from build123d import *

# Parameters (mm, degrees)
BOSS_EXTRUDE1_DEPTH = 1219.2
SKETCH3_R           = 4.7625
CUT_EXTRUDE1_DEPTH  = 1.27
SKETCH4_R           = 4.7625
CUT_EXTRUDE2_DEPTH  = 1.27
FILLET1_R           = 3.175
FILLET2_R           = 1.5875
CUT_EXTRUDE3_DEPTH  = 457.2


with BuildPart() as part:
    # Sketch1 → Boss-Extrude1 (new body)
    with BuildSketch(Plane(origin=(0, 0, 0), x_dir=(1, 0, 0), z_dir=(0, 1, 0))):
        Polygon((1.27, 1.27), (1.27, 30.48), (1.27, 31.75), (0, 31.75), (0, 0), (31.75, 0), (31.75, 1.27), (30.48, 1.27), align=None)
    extrude(amount=BOSS_EXTRUDE1_DEPTH)

    # Sketch3 → Cut-Extrude1 (cut)
    with BuildSketch(Plane.ZY):
        with Locations((-17.4625, 12.7)):
            Circle(SKETCH3_R)
        with Locations((-17.4625, 38.1)):
            Circle(SKETCH3_R)
        with Locations((-17.4625, 63.5)):
            Circle(SKETCH3_R)
        with Locations((-17.4625, 88.9)):
            Circle(SKETCH3_R)
        with Locations((-17.4625, 114.3)):
            Circle(SKETCH3_R)
        with Locations((-17.4625, 139.7)):
            Circle(SKETCH3_R)
        with Locations((-17.4625, 165.1)):
            Circle(SKETCH3_R)
        with Locations((-17.4625, 190.5)):
            Circle(SKETCH3_R)
        with Locations((-17.4625, 215.9)):
            Circle(SKETCH3_R)
        with Locations((-17.4625, 241.3)):
            Circle(SKETCH3_R)
        with Locations((-17.4625, 266.7)):
            Circle(SKETCH3_R)
        with Locations((-17.4625, 292.1)):
            Circle(SKETCH3_R)
        with Locations((-17.4625, 317.5)):
            Circle(SKETCH3_R)
        with Locations((-17.4625, 342.9)):
            Circle(SKETCH3_R)
        with Locations((-17.4625, 368.3)):
            Circle(SKETCH3_R)
        with Locations((-17.4625, 393.7)):
            Circle(SKETCH3_R)
        with Locations((-17.4625, 419.1)):
            Circle(SKETCH3_R)
        with Locations((-17.4625, 444.5)):
            Circle(SKETCH3_R)
        with Locations((-17.4625, 469.9)):
            Circle(SKETCH3_R)
        with Locations((-17.4625, 495.3)):
            Circle(SKETCH3_R)
        with Locations((-17.4625, 520.7)):
            Circle(SKETCH3_R)
        with Locations((-17.4625, 546.1)):
            Circle(SKETCH3_R)
        with Locations((-17.4625, 571.5)):
            Circle(SKETCH3_R)
        with Locations((-17.4625, 596.9)):
            Circle(SKETCH3_R)
        with Locations((-17.4625, 622.3)):
            Circle(SKETCH3_R)
        with Locations((-17.4625, 647.7)):
            Circle(SKETCH3_R)
        with Locations((-17.4625, 673.1)):
            Circle(SKETCH3_R)
        with Locations((-17.4625, 698.5)):
            Circle(SKETCH3_R)
        with Locations((-17.4625, 723.9)):
            Circle(SKETCH3_R)
        with Locations((-17.4625, 749.3)):
            Circle(SKETCH3_R)
        with Locations((-17.4625, 774.7)):
            Circle(SKETCH3_R)
        with Locations((-17.4625, 800.1)):
            Circle(SKETCH3_R)
        with Locations((-17.4625, 825.5)):
            Circle(SKETCH3_R)
        with Locations((-17.4625, 850.9)):
            Circle(SKETCH3_R)
        with Locations((-17.4625, 876.3)):
            Circle(SKETCH3_R)
        with Locations((-17.4625, 901.7)):
            Circle(SKETCH3_R)
        with Locations((-17.4625, 927.1)):
            Circle(SKETCH3_R)
        with Locations((-17.4625, 952.5)):
            Circle(SKETCH3_R)
        with Locations((-17.4625, 977.9)):
            Circle(SKETCH3_R)
        with Locations((-17.4625, 1003.3)):
            Circle(SKETCH3_R)
        with Locations((-17.4625, 1028.7)):
            Circle(SKETCH3_R)
        with Locations((-17.4625, 1054.1)):
            Circle(SKETCH3_R)
        with Locations((-17.4625, 1079.5)):
            Circle(SKETCH3_R)
        with Locations((-17.4625, 1104.9)):
            Circle(SKETCH3_R)
        with Locations((-17.4625, 1130.3)):
            Circle(SKETCH3_R)
        with Locations((-17.4625, 1155.7)):
            Circle(SKETCH3_R)
        with Locations((-17.4625, 1181.1)):
            Circle(SKETCH3_R)
        with Locations((-17.4625, 1206.5)):
            Circle(SKETCH3_R)
    extrude(amount=-CUT_EXTRUDE1_DEPTH, mode=Mode.SUBTRACT)

    # Sketch4 → Cut-Extrude2 (cut)
    with BuildSketch(Plane.XY):
        with Locations((17.4625, 1206.5)):
            Circle(SKETCH4_R)
        with Locations((17.4625, 1181.1)):
            Circle(SKETCH4_R)
        with Locations((17.4625, 1155.7)):
            Circle(SKETCH4_R)
        with Locations((17.4625, 1130.3)):
            Circle(SKETCH4_R)
        with Locations((17.4625, 1104.9)):
            Circle(SKETCH4_R)
        with Locations((17.4625, 1079.5)):
            Circle(SKETCH4_R)
        with Locations((17.4625, 1054.1)):
            Circle(SKETCH4_R)
        with Locations((17.4625, 1028.7)):
            Circle(SKETCH4_R)
        with Locations((17.4625, 1003.3)):
            Circle(SKETCH4_R)
        with Locations((17.4625, 977.9)):
            Circle(SKETCH4_R)
        with Locations((17.4625, 952.5)):
            Circle(SKETCH4_R)
        with Locations((17.4625, 927.1)):
            Circle(SKETCH4_R)
        with Locations((17.4625, 901.7)):
            Circle(SKETCH4_R)
        with Locations((17.4625, 876.3)):
            Circle(SKETCH4_R)
        with Locations((17.4625, 850.9)):
            Circle(SKETCH4_R)
        with Locations((17.4625, 825.5)):
            Circle(SKETCH4_R)
        with Locations((17.4625, 800.1)):
            Circle(SKETCH4_R)
        with Locations((17.4625, 774.7)):
            Circle(SKETCH4_R)
        with Locations((17.4625, 749.3)):
            Circle(SKETCH4_R)
        with Locations((17.4625, 723.9)):
            Circle(SKETCH4_R)
        with Locations((17.4625, 698.5)):
            Circle(SKETCH4_R)
        with Locations((17.4625, 673.1)):
            Circle(SKETCH4_R)
        with Locations((17.4625, 647.7)):
            Circle(SKETCH4_R)
        with Locations((17.4625, 622.3)):
            Circle(SKETCH4_R)
        with Locations((17.4625, 596.9)):
            Circle(SKETCH4_R)
        with Locations((17.4625, 571.5)):
            Circle(SKETCH4_R)
        with Locations((17.4625, 546.1)):
            Circle(SKETCH4_R)
        with Locations((17.4625, 520.7)):
            Circle(SKETCH4_R)
        with Locations((17.4625, 495.3)):
            Circle(SKETCH4_R)
        with Locations((17.4625, 469.9)):
            Circle(SKETCH4_R)
        with Locations((17.4625, 444.5)):
            Circle(SKETCH4_R)
        with Locations((17.4625, 419.1)):
            Circle(SKETCH4_R)
        with Locations((17.4625, 393.7)):
            Circle(SKETCH4_R)
        with Locations((17.4625, 368.3)):
            Circle(SKETCH4_R)
        with Locations((17.4625, 342.9)):
            Circle(SKETCH4_R)
        with Locations((17.4625, 317.5)):
            Circle(SKETCH4_R)
        with Locations((17.4625, 292.1)):
            Circle(SKETCH4_R)
        with Locations((17.4625, 266.7)):
            Circle(SKETCH4_R)
        with Locations((17.4625, 241.3)):
            Circle(SKETCH4_R)
        with Locations((17.4625, 215.9)):
            Circle(SKETCH4_R)
        with Locations((17.4625, 190.5)):
            Circle(SKETCH4_R)
        with Locations((17.4625, 165.1)):
            Circle(SKETCH4_R)
        with Locations((17.4625, 139.7)):
            Circle(SKETCH4_R)
        with Locations((17.4625, 114.3)):
            Circle(SKETCH4_R)
        with Locations((17.4625, 88.9)):
            Circle(SKETCH4_R)
        with Locations((17.4625, 63.5)):
            Circle(SKETCH4_R)
        with Locations((17.4625, 38.1)):
            Circle(SKETCH4_R)
        with Locations((17.4625, 12.7)):
            Circle(SKETCH4_R)
    extrude(amount=-CUT_EXTRUDE2_DEPTH, mode=Mode.SUBTRACT)

    # Fillet1
    fillet1_edges = [part.edges().sort_by_distance(p)[0] for p in [
        (0, 609.6, 0),
    ]]
    fillet(fillet1_edges, radius=FILLET1_R)

    # Fillet2
    fillet2_edges = [part.edges().sort_by_distance(p)[0] for p in [
        (1.27, 609.6, -1.27),
    ]]
    fillet(fillet2_edges, radius=FILLET2_R)

    # Sketch5 → Cut-Extrude3 (cut)
    with BuildSketch(Plane(origin=(0, 1219.2, 0), x_dir=(1, 0, 0), z_dir=(0, 1, 0))):
        with BuildLine():
            Line((0, 31.75), (0, 3.175))
            ThreePointArc((0, 3.175), (0.92993597, 0.92993597), (3.175, 0))
            Line((3.175, 0), (31.75, 0))
            Line((31.75, 0), (31.75, 1.27))
            Line((31.75, 1.27), (2.8575, 1.27))
            ThreePointArc((2.8575, 1.27), (1.734967985, 1.734967985), (1.27, 2.8575))
            Line((1.27, 2.8575), (1.27, 31.75))
            Line((1.27, 31.75), (0, 31.75))
        make_face()
    extrude(amount=-CUT_EXTRUDE3_DEPTH, mode=Mode.SUBTRACT)


solid = part.part
The listing builds one solid part. Answer for the finished solid, in the listing's coordinates (mm). A direction names the side the tool comes from. Give positions to 0.01 mm unless a question says otherwise; leave off trailing zeros.
1) A tool of negligible diameter and unlimited length cuts with its end or side. For faces 1 (the face through (1.27, 376, -17)), 2 (the face through (0, 376, -18)), from which of +Z, -Z, +X, -X, +Y, -Y can it reach the whole face along a straight path? Write none if from no direction.
2) Find the intervals of material crossed by L1, parallel to Z at x = 0.7, y = 393.7 (3 decimals); L2, parallel to Z at x = 19.5, y = 512.5; L3, parallel to X at y = 136.5, z = -29, in increasing order.
3) Given P1, Ø11, axis at y = 317.5, z = -17.46, coming from the +X side; P2, Ø5.5, axis at y = 266.7, z = -17.46, coming from the -X side (1 decimal); P3, Ø1, axis at x = 22, y = 381.5, coming from the -Z side, each flat-ended and moving along its own axis, determine where each tip first touches the part or whether it passes through.
Response:
1. face 1: -Z, +X, +Y, -Y
1. face 2: +Z, -Z, -X, +Y, -Y
2. L1: z = -31.75 to -22.225, -12.7 to -1.186
2. L2: z = -1.27 to 0
2. L3: x = 0 to 1.27
3. P1: stops at x = 1.27
3. P2: passes through
3. P3: stops at z = -1.27
